Design review of the part built by this model. Coordinates are the model's own, in mm. Coordinates: 2 decimals unless noted, no trailing zeros. Order: outer loops, then holes, each group sorted by start corner. A loop starts at its lowest first (then second) coordinate and runs counter-clockwise, first axis right, second up. Notation, with made-up numbers: M 70,20 L 89,20 A16 ccw 89,33 Z; hole C -37,41.25 d10. An arc over 180 degrees is marked long. Answer in a Markdown table with one row per item.
from build123d import *

# Parameters (mm, degrees)
SKETCH1_W           = 406.4
SKETCH1_H           = 25.4
SKETCH1_R           = 6.35
SKETCH1_R_2         = 2.5796875
BOSS_EXTRUDE1_DEPTH = 2.38125
FILLET1_R           = 6.35


with BuildPart() as part:
    # Sketch1 → Boss-Extrude1 (new body)
    with BuildSketch(Plane(origin=(0, 0, 0), x_dir=(1, 0, 0), z_dir=(0, 1, 0))):
        with Locations((203.2, 12.7)):
            Rectangle(SKETCH1_W, SKETCH1_H)
        with Locations(Location((12.7, 12.7, 0), (0, 0, 90))):
            Circle(SKETCH1_R, mode=Mode.SUBTRACT)
        with Locations(Location((393.7, 12.7, 0), (0, 0, 90))):
            Circle(SKETCH1_R, mode=Mode.SUBTRACT)
        with Locations(Location((139.7, 12.7, 0), (0, 0, 90))):
            Circle(SKETCH1_R, mode=Mode.SUBTRACT)
        with Locations(Location((266.7, 12.7, 0), (0, 0, 90))):
            Circle(SKETCH1_R, mode=Mode.SUBTRACT)
        with Locations(Location((76.2, 12.7, 0), (0, 0, 90))):
            Circle(SKETCH1_R_2, mode=Mode.SUBTRACT)
        with Locations(Location((203.2, 12.7, 0), (0, 0, 90))):
            Circle(SKETCH1_R_2, mode=Mode.SUBTRACT)
        with Locations(Location((330.2, 12.7, 0), (0, 0, 90))):
            Circle(SKETCH1_R_2, mode=Mode.SUBTRACT)
    extrude(amount=BOSS_EXTRUDE1_DEPTH)

    # Fillet1
    fillet1_edges = [part.edges().sort_by_distance(p)[0] for p in [
        (0, 1.190625, -25.4),
        (406.4, 1.190625, -25.4),
        (406.4, 1.190625, 0),
        (0, 1.190625, 0),
    ]]
    fillet(fillet1_edges, radius=FILLET1_R)


solid = part.part
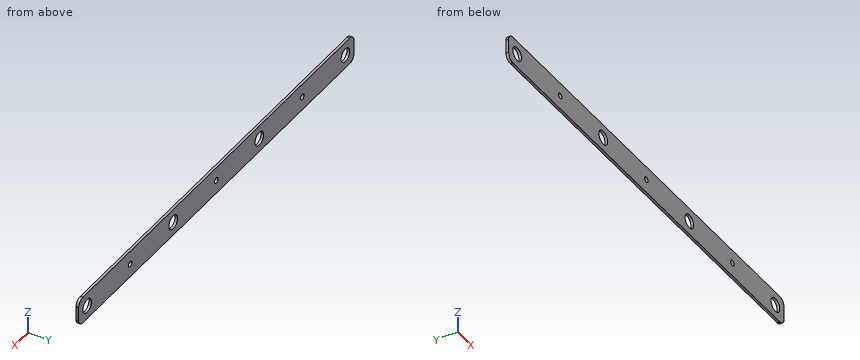
(1) Insertion check: pin 1 Ø5 at (x, z) = (295.5, -6.5) entering from -Y. The pin has a flat end and moves straight along its axis. Give the tip position at first contact, or say it passes through.
Return value:
| item | result |
|---|---|
| pin 1 | stops at y = 0 |
(2) Add section B-B, the plane x = 393.7. Give the boundary of the cut face in (y, z).
Return value:
| item | result |
|---|---|
| outline | M 0,-25.4 L 2.38,-25.4 L 2.38,-19.05 L 0,-19.05 Z; M 0,-6.35 L 2.38,-6.35 L 2.38,0 L 0,0 Z |
(3) Add section A-A, the plane y = 1.2. Give the boundary of the cut face in (x, z), and give its area (3 significant figures).
Return value:
| item | result |
|---|---|
| outline | M 0,-19.05 A6.35 ccw 6.35,-25.4 L 400.05,-25.4 A6.35 ccw 406.4,-19.05 L 406.4,-6.35 A6.35 ccw 400.05,0 L 6.35,0 A6.35 ccw 0,-6.35 Z; hole C 12.7,-12.7 d12.7; hole C 76.2,-12.7 d5.16; hole C 139.7,-12.7 d12.7; hole C 203.2,-12.7 d5.16; hole C 266.7,-12.7 d12.7; hole C 330.2,-12.7 d5.16; hole C 393.7,-12.7 d12.7 |
| area | 9,720 mm2 |
(4) For line 1 along Z through (x, y) = (393.7, 1.75); line 2 along Z through (x, y) = (330.2, 0.5); line 3 along X through (y, z) = (1.55, -8), list the stretches that pass through material, from the lowest coordinate up. Write a range as from..to.
Return value:
| item | result |
|---|---|
| line 1 | z = -25.4..-19.05, -6.35..0 |
| line 2 | z = -25.4..-15.28, -10.12..0 |
| line 3 | x = 0..8.43, 16.97..135.43, 143.97..262.43, 270.97..389.43, 397.97..406.4 |
